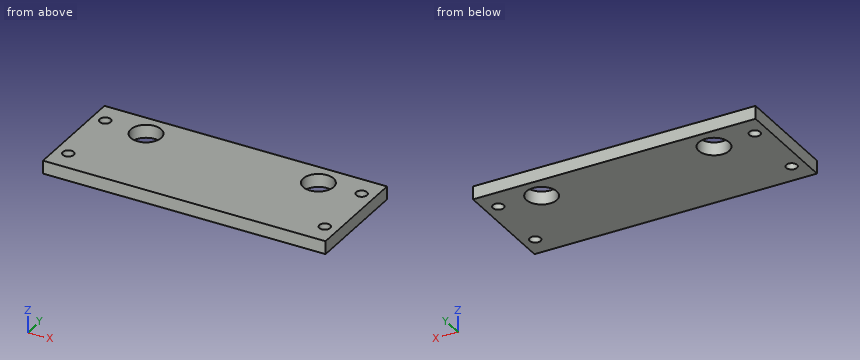
from build123d import *

# Parameters (mm, degrees)
SKETCH_1_W      = 65
SKETCH_1_H      = 25
SKETCH_1_R      = 3.5
EXTRUDE_1_DEPTH = 3
M3X0_5_1_D      = 2.5
M3X0_5_1_DEPTH  = 8.5
M3X0_5_1_TIP    = 0.751075774


with BuildPart() as part:
    # ｽｹｯﾁ1 → ﾎﾞｽ - 押し出し1 (new body)
    with BuildSketch(Plane.XY):
        Rectangle(SKETCH_1_W, SKETCH_1_H)
        with Locations((-19.83, 7)):
            Circle(SKETCH_1_R, mode=Mode.SUBTRACT)
        with Locations((19.83, 7)):
            Circle(SKETCH_1_R, mode=Mode.SUBTRACT)
    extrude(amount=EXTRUDE_1_DEPTH)

    # M3x0.5 ねじ穴1
    with Locations(Plane(origin=(-29.5, 7.5, 3), x_dir=(1, 0, 0), z_dir=(0, 0, 1))):
        with Locations((0, 0), (0, -15), (59, 0), (59, -15)):
            Hole(M3X0_5_1_D / 2, depth=M3X0_5_1_DEPTH)
            with Locations((0, 0, -(M3X0_5_1_DEPTH + M3X0_5_1_TIP / 2))):  # 118° drill point
                Cone(0, M3X0_5_1_D / 2, M3X0_5_1_TIP, mode=Mode.SUBTRACT)


solid = part.part
Can you work these out from the model? Positions are in its coordinate system, mm. Coordinates: 2 decimals unless noted, no trailing zeros. Order: outer loops, then holes, each group sorted by start corner. A loop starts at its lowest first (then second) coordinate and runs counter-clockwise, first axis right, second up. Notation, with made-up numbers: (-2, 31) - (57, 31) arc R9 cw to (57, 42) - close; hole circle Ø2 at (-13.5, 56.5). An arc over 180 degrees is marked (long way). Answer as a JSON object with one key per item and string values. Group by question number.
Q1. I need wall thicknesses on line 1 (Y direction, x = -20, z = 0.8); line 2 (X direction, y = -6.75, z = 1.25); line 3 (Y direction, x = 28.5, z = 2.1). Which ranges of each line are inside material? Lowest first, please. Write a range as from..to.
Q2. Imagine slicing it at C-C (z = 1.4). Please give me the cut outline in (x, y), and give its area (3 significant figures).
Q3. Imagine slicing it at A-A (x = -29.5). Please give me the cut outline in (y, z).
Q4. Will this pin go through, and if not, where does the flat tip stop? P1, Ø2, axis at x = 29.5, y = -7.5, coming from the +Z side.
Q5. Imagine slicing it at B-B (y = -7.5). Please give me the cut outline in (x, z).
Q6. Imagine slicing it at D-D (x = -19.83). Please give me the cut outline in (y, z), and give its area (3 significant figures).
Determined:
{
 "1": {"line 1": "y = -12.5..3.5, 10.5..12.5", "line 2": "x = -32.5..-30.5, -28.5..28.5, 30.5..32.5", "line 3": "y = -12.5..-8.25, -6.75..6.75, 8.25..12.5"},
 "2": {"outline": "(-32.5, -12.5) - (32.5, -12.5) - (32.5, 12.5) - (-32.5, 12.5) - close; hole circle Ø2.5 at (-29.5, -7.5); hole circle Ø2.5 at (-29.5, 7.5); hole circle Ø7 at (-19.83, 7); hole circle Ø7 at (19.83, 7); hole circle Ø2.5 at (29.5, -7.5); hole circle Ø2.5 at (29.5, 7.5)", "area": "1,530 mm2"},
 "3": {"outline": "(-12.5, 0) - (-8.75, 0) - (-8.75, 3) - (-12.5, 3) - close; (-6.25, 0) - (6.25, 0) - (6.25, 3) - (-6.25, 3) - close; (8.75, 0) - (12.5, 0) - (12.5, 3) - (8.75, 3) - close"},
 "4": {"P1": "passes through"},
 "5": {"outline": "(-32.5, 0) - (-30.75, 0) - (-30.75, 3) - (-32.5, 3) - close; (-28.25, 0) - (28.25, 0) - (28.25, 3) - (-28.25, 3) - close; (30.75, 0) - (32.5, 0) - (32.5, 3) - (30.75, 3) - close"},
 "6": {"outline": "(-12.5, 0) - (3.5, 0) - (3.5, 3) - (-12.5, 3) - close; (10.5, 0) - (12.5, 0) - (12.5, 3) - (10.5, 3) - close", "area": "54.0 mm2"}
}
